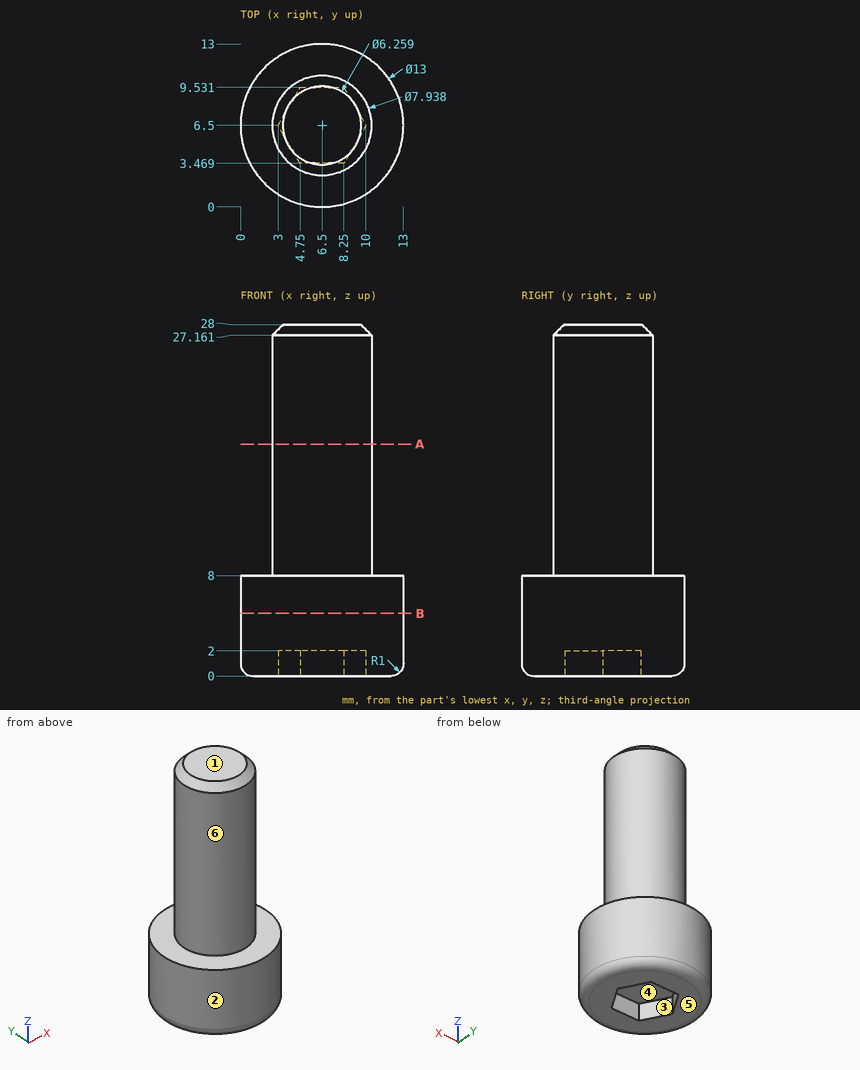
Geometry: see drawing. Coordinates: mm, zero at the bounding-box minimum. A direction names the side the tool comes from. Coordinates: 2 decimals unless noted, no trailing zeros. Order: outer loops, then holes, each group sorted by start corner. A loop starts at its lowest first (then second) coordinate and runs counter-clockwise, first axis right, second up. Notation, with made-up numbers: M 19.25,1.25 L 35.25,1.25 A13 ccw 35.25,7.25 Z; hole C 31.5,9 d10. An arc over 180 degrees is marked long. Answer in a Markdown table with one row per item. Add a question column.
Q1. Mould query, pull axis X, two halves, no side actions, for the marked faces 1, 2, 3 and 4. Classes: released by +X, released by -X, zero draft, split by the parting line, or undercut.
Q2. Section query A-A on z = 18.5. Return the cut outline in (x, y).
Q3. Reachability of the marked faces 5 and 6 from +Z, -Z, +X, -X, +Y, -Y: full face, straight path, thin tool, end or side. Return the list, or none.
Q4. Section query B-B on z = 5. Return the cut outline in (x, y), and give its area (3 significant figures).
Q5. Contact query for flat-ended pins moving along their axis: P1, Ø3, axis at x = 7.5, y = 7, coming from the -Z side; P2, Ø5, axis at x = 8, z = 18.5, coming from the +Y side; P3, Ø4, axis at x = 11, z = 23, coming from the +Y side. Output: stop coordinate, or through.
Q6. Line query: L1, parallel to Z at x = 8.75, y = 7.25; L2, parallel to Z at x = 3, y = 2.75; L3, parallel to Y at x = 8.25, z = 12.75. Output: solid intervals per line, ascending.
Completed:
| question | item | result |
|---|---|---|
| 1 | face 1 | zero draft |
| 1 | face 2 | split by the parting line |
| 1 | face 3 | undercut |
| 1 | face 4 | undercut |
| 2 | outline | C 6.5,6.5 d7.94 |
| 3 | face 5 | -Z, +X, -X, +Y, -Y |
| 3 | face 6 | +Z |
| 4 | outline | C 6.5,6.5 d13 |
| 4 | area | 133 mm2 |
| 5 | P1 | stops at z = 2 |
| 5 | P2 | stops at y = 10.47 |
| 5 | P3 | stops at y = 9.58 |
| 6 | L1 | z = 2 to 28 |
| 6 | L2 | z = 0 to 8 |
| 6 | L3 | y = 2.94 to 10.06 |
